from build123d import *

# Parameters (mm, degrees)
F0_R     = 11.2
F1_DEPTH = 2.4


with BuildPart() as f1:
    # F0 (on Top) → F1 (new body)
    with BuildSketch(Plane.XY):
        with BuildLine():
            ThreePointArc((11.314053, 6.446049), (9.351579, 13.010427), (10.577312, 19.751342))
            ThreePointArc((10.577312, 19.751342), (-0.177298, 39.479362), (-10.376945, 19.458782))
            ThreePointArc((-10.376945, 19.458782), (-11.356072, 6.375934), (-22.39382, -0.71545))
            ThreePointArc((-22.39382, -0.71545), (-34.101481, -19.893226), (-11.663327, -18.716089))
            ThreePointArc((-11.663327, -18.716089), (0.156315, -13.022614), (11.816508, -19.035892))
            ThreePointArc((11.816508, -19.035892), (34.27878, -19.586136), (22.040272, -0.742693))
            ThreePointArc((22.040272, -0.742693), (15.845674, 1.611026), (11.314053, 6.446049))
        make_face()
        with Locations((-23.19268, -13.3903)):
            Circle(F0_R, mode=Mode.SUBTRACT)
        with Locations((23.19268, -13.3903)):
            Circle(F0_R, mode=Mode.SUBTRACT)
        Circle(F0_R, mode=Mode.SUBTRACT)
        with Locations((0, 26.7806)):
            Circle(F0_R, mode=Mode.SUBTRACT)
    extrude(amount=F1_DEPTH)


solid = f1.part
Could you check a few things on this model? Use its own coordinates, in mm. Give positions to 0.01 mm unless a question says otherwise; leave off trailing zeros. Order: outer loops, then holes, each group sorted by start corner. A loop starts at its lowest first (then second) coordinate and runs counter-clockwise, first axis right, second up. Notation, with made-up numbers: (23.5, 44.25) - (44.5, 44.25) arc R14 ccw to (44.5, 49.25) - close; hole circle Ø7 at (10, 70.5). An arc over 180 degrees is marked (long way). One line per item, written item: value. Start each with the question number.
1. Imagine slicing it at B-B on y = -17. List the corners of the cut face in (x, z) for me, plus the area to 3 significant figures.
2. Thinking about a two-plate mould opening in X: for faces 1 (the face through (-5.5, -10.2, 0)), 2 (the face through (-12.847, -17.68, 1.183)), 3 (the face through (-11.26, 6.54, 1.18)), which applies, +X half, -X half, draft (parallel to the pull), parting line (faces both ways), or undercut?
3. Imagine slicing it at D-D on x = 2.5. List the corners of the cut face in (y, z) for me.
4. Imagine slicing it at A-A on x = -14.5. List the corners of the cut face in (y, z) for me.
5. Imagine slicing it at C-C on y = 17.5. List the corners of the cut face in (x, z) for me.
6. If I drill on probe 1 along Y at (x, z) = (-0.5, 1.1); probe 2 along X at (y, z) = (-7, 2.1); probe 3 along X at (y, z) = (-22, 2.1), over which ranges is the centre line in solid material (lowest first)?
7. For P1, Ø1, axis at y = 28, z = 2, coming from the +X side; P2, Ø3, axis at x = -15.5, y = -7, coming from the +Z side; P3, Ø1, axis at x = 26, z = 2, coming from the +Y side, each with a flat end and sliding along its axis, tell me the tip position at first contact or that it passes through.
Values:
1. outline: (-35.37, 0) - (-33.8, 0) - (-33.8, 2.4) - (-35.37, 2.4) - close; (-12.59, 0) - (-10.1, 0) - (-10.1, 2.4) - (-12.59, 2.4) - close; (10.01, 0) - (12.59, 0) - (12.59, 2.4) - (10.01, 2.4) - close; (33.8, 0) - (35.37, 0) - (35.37, 2.4) - (33.8, 2.4) - close
1. area: 19.7 mm²
2. face 1: draft
2. face 2: undercut
2. face 3: -X half
3. outline: (-13.24, 0) - (-10.92, 0) - (-10.92, 2.4) - (-13.24, 2.4) - close; (10.92, 0) - (15.86, 0) - (15.86, 2.4) - (10.92, 2.4) - close; (37.7, 0) - (39.23, 0) - (39.23, 2.4) - (37.7, 2.4) - close
4. outline: (-22.65, 0) - (-20.45, 0) - (-20.45, 2.4) - (-22.65, 2.4) - close; (-6.33, 0) - (2.67, 0) - (2.67, 2.4) - (-6.33, 2.4) - close
5. outline: (-9.73, 0) - (-6.27, 0) - (-6.27, 2.4) - (-9.73, 2.4) - close; (6.27, 0) - (9.8, 0) - (9.8, 2.4) - (6.27, 2.4) - close
6. probe 1: -13.03 to -11.19, 11.19 to 15.59, 37.97 to 39.47
6. probe 2: -34.17 to -32.39, -13.99 to -8.74, 8.74 to 13.99, 32.39 to 34.17
6. probe 3: -32.53 to -30.36, -16.03 to -13.86, 13.86 to 16.03, 30.36 to 32.53
7. P1: x = 12.68
7. P2: z = 2.4
7. P3: y = -0.9
